The figure shows three views and two pictorial views of one solid part (mm, origin at its lowest corner). Answer the questions. A direction names the side the tool comes from. Coordinates: 2 decimals unless noted, no trailing zeros. Write each loop counter-clockwise with the first axis right and the second up, starting at its lowest first coordinate (ties: lowest second). Pieces come first, ordered by that corner, then holes. Notation, with made-up numbers: M 40.5,19.5 L 51.5,19.5 A22 cw 51.5,49.5 Z; hole C 78.5,38.5 d11. An arc over 180 degrees is marked long. Use CSV: the item, a comma, the result in double quotes.
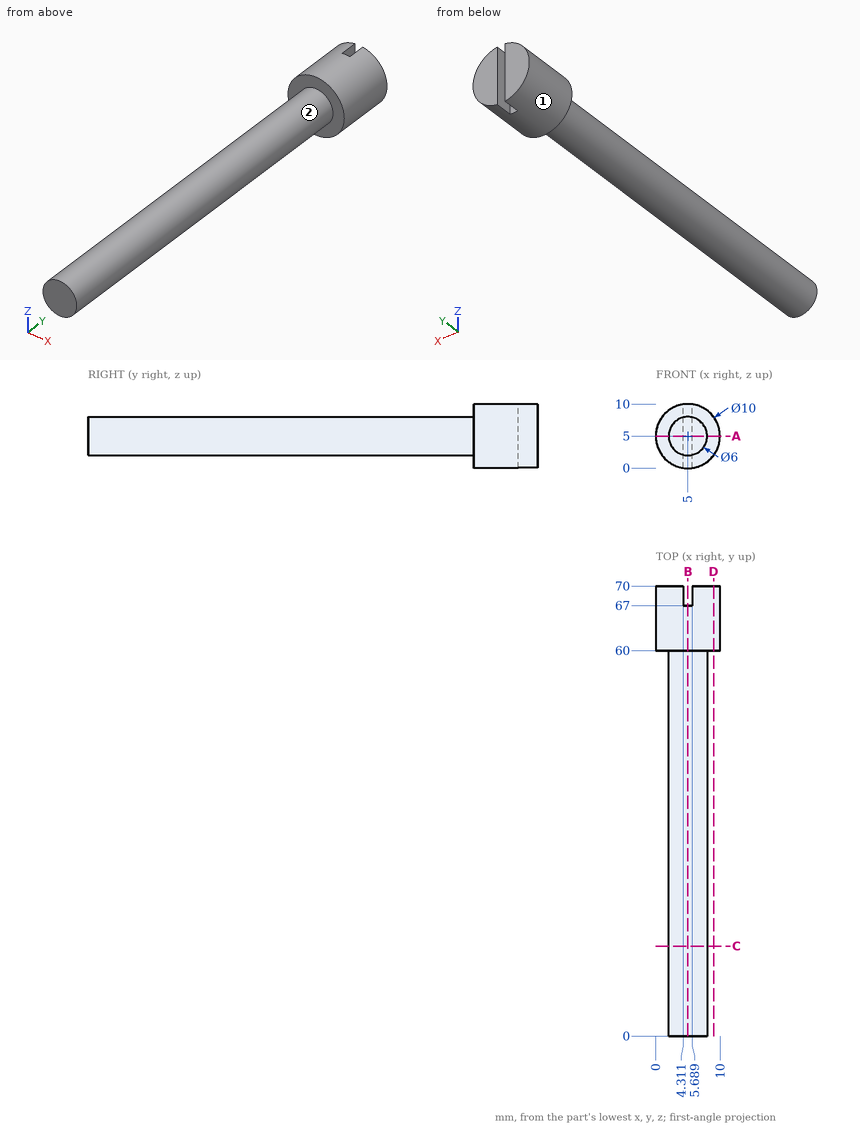
Item 1: The part is cut by section C-C (y = 14). Write down the section's boundary in (x, z), then the cut area to 3 significant figures.
Answer:
outline,"C 5,5 d6"
area,"28.3 mm2"
Item 2: Consider probe 1 along Y at (x, z) = (5.5, 4.75); probe 2 along Z at (x, y) = (4.75, 9.5); probe 3 along Y at (x, z) = (4, 9.5). Determine where each line is inside the solid, lowest interval first.
Answer:
probe 1,"y = 0 to 67"
probe 2,"z = 2.01 to 7.99"
probe 3,"y = 60 to 70"
Item 3: Given pin 1 (1.5 mm diameter, centred on y = 21, z = 2, fed in from +X); pin 2 (3 mm diameter, centred on x = 7, y = 16, fed in from -Z); pin 3 (2 mm diameter, centred on y = 37.5, z = 3, fed in from -X), each flat-ended and moving along its own axis, determine where each tip first touches the part or whether it passes through.
Answer:
pin 1,"stops at x = 6.98"
pin 2,"stops at z = 2.04"
pin 3,"stops at x = 2.17"
Item 4: The part is cut by section B-B (x = 5). Write down the section's boundary in (y, z), then the cut area to 3 significant figures.
Answer:
outline,"M 0,2 L 60,2 L 60,0 L 67,0 L 67,10 L 60,10 L 60,8 L 0,8 Z"
area,"430 mm2"
Item 5: The part is cut by section D-D (x = 9). Write down the section's boundary in (y, z).
Answer:
outline,"M 60,2 L 70,2 L 70,8 L 60,8 Z"
Item 6: The part is cut by section A-A (z = 5). Write down the section's boundary in (x, y), then the cut area to 3 significant figures.
Answer:
outline,"M 0,60 L 2,60 L 2,0 L 8,0 L 8,60 L 10,60 L 10,70 L 5.69,70 L 5.69,67 L 4.31,67 L 4.31,70 L 0,70 Z"
area,"456 mm2"
Item 7: A tool of negligible diameter and unlimited length cuts with its end or side. For the marked faces 1 and 2, from which of +Z, -Z, +X, -X, +Y, -Y can it reach the whole face along a straight path? Write none if from no direction.
Answer:
face 1,"+Y, -Y"
face 2,"-Y"
